Part model, mm, in its own coordinate system. A direction names the side the tool comes from. Coordinates: 2 decimals unless noted, no trailing zeros. Order: outer loops, then holes, each group sorted by start corner. A loop starts at its lowest first (then second) coordinate and runs counter-clockwise, first axis right, second up. Notation, with made-up numbers: M 75.5,6 L 90.5,6 A19 ccw 90.5,19 Z; hole C 28,-36 d2. An arc over 180 degrees is marked long. Answer in a Markdown table with one row per item. Add a question column.
from build123d import *

# Parameters (mm, degrees)
SKETCH1_W                     = 64.008
SKETCH1_H                     = 24.9936
BOSS_EXTRUDE1_DEPTH           = 6.35
SKETCH2_W                     = 64.008
SKETCH2_H                     = 6.35
BOSS_EXTRUDE2_DEPTH           = 82.55
CBORE_FOR_M5_SHCS1_AT_2_COUNT = 2
CBORE_FOR_M5_SHCS1_AT_2_PITCH = 50
SKETCH8_W                     = 10.414
SKETCH8_H                     = 82.55
CUT_EXTRUDE1_DEPTH            = 112.120735621
SKETCH9_W                     = 3.048
SKETCH9_H                     = 82.55
CUT_EXTRUDE3_DEPTH            = 112.120735621


with BuildPart() as part:
    # Sketch1 → Boss-Extrude1 (new body)
    with BuildSketch(Plane.XY):
        with Locations((32.004, 12.4968)):
            Rectangle(SKETCH1_W, SKETCH1_H)
    extrude(amount=BOSS_EXTRUDE1_DEPTH)

    # Sketch2 → Boss-Extrude2 (add)
    with BuildSketch(Plane.XY.offset(6.35)):
        with Locations((32.004, 3.175)):
            Rectangle(SKETCH2_W, SKETCH2_H)
    extrude(amount=BOSS_EXTRUDE2_DEPTH)

    # Sketch7 → CBORE for M5 SHCS1 (revolve, cut)
    with BuildSketch(Plane(origin=(7, 12.5, 6.35), x_dir=(0, -1, 0), z_dir=(1, 0, 0))):
        Polygon((0, 0), (0, 6.35), (2.75, 6.35), (2.75, 5), (5, 5), (5, 0.025), (5.025, 0), align=None)
    cbore_for_m5_shcs1 = revolve(axis=Axis((7, 12.5, 12.7), (0, 0, -1)), mode=Mode.SUBTRACT)

    # CBORE for M5 SHCS1 at 2: CBORE for M5 SHCS1 ×2
    with Locations(*[(i * CBORE_FOR_M5_SHCS1_AT_2_PITCH, 0, 0) for i in range(1, CBORE_FOR_M5_SHCS1_AT_2_COUNT)]):
        add(cbore_for_m5_shcs1, mode=Mode.SUBTRACT)

    # Sketch8 → Cut-Extrude1 (cut, through all)
    with BuildSketch(Plane(origin=(0, 6.35, 0), x_dir=(1, 0, 0), z_dir=(0, 1, 0))):
        with Locations((5.207, -47.625)):
            Rectangle(SKETCH8_W, SKETCH8_H)
    extrude(amount=-CUT_EXTRUDE1_DEPTH, mode=Mode.SUBTRACT)

    # Sketch9 → Cut-Extrude3 (cut, through all)
    with BuildSketch(Plane(origin=(0, 6.35, 0), x_dir=(1, 0, 0), z_dir=(0, 1, 0))):
        with Locations((62.484, -47.625)):
            Rectangle(SKETCH9_W, SKETCH9_H)
    extrude(amount=-CUT_EXTRUDE3_DEPTH, mode=Mode.SUBTRACT)


solid = part.part
(1) Slice it at D-D (x = 7). List the corners of the cut face in (y, z) (3 decimals).
(2) Slice it at B-B (y = 12.5). List the corners of the cut face in (x, z) (3 decimals), and give its area (3 significant figures).
(3) Pull direction Y, two halves, no side cores. Call faces 5 (the flat face through (39, 0, 44)), 6 (the cylindrical face through (52.784, 9.812, 3.872)), 7 (the flat face through (0, 12, 3)): pulls with the +Y half, pulls with the -Y half, needs draft (parallel to the pull), parting line crosses it, or undercut.
(4) 3-axis set-ups, long thin cutter, end or side, ignore diameter. For faces 1 (the flat face through (35, 6.35, 47)), 2 (the flat face through (60.96, 3, 48)), 3 (the flat face through (10.414, 3, 48)), 4 (the cylindrical face through (5.5, 7.73, 3.87)): which of +Z, -Z, +X, -X, +Y, -Y reach the whole face in a straight line?
(5) Wall check: line 1 (X direction, y = 12.5, z = 3.85); line 2 (X direction, y = 12.5, z = 0.85); line 3 (Y direction, x = 7, z = 4). Give the ranges that are in metal, low to high.
(6) Drop flat-ended pins along their axis: P1, Ø5, axis at x = 10, y = 13, coming from the -Z side; P2, Ø6, axis at x = 57, y = 12.5, coming from the +Z side; P3, Ø7, axis at y = 2.5, z = 39.5, coming from the +X side; P4, Ø8, axis at x = 5.5, y = 14.5, coming from the +Z side. Give the stop position or say it passes through.
(7) Slice it at A-A (x = 57). List the corners of the cut face in (y, z) (3 decimals).
(8) Slice it at C-C (y = 3.5). List the corners of the cut face in (x, z).
Computed:
| question | item | result |
|---|---|---|
| 1 | outline | M 0,0 L 9.75,0 L 9.75,1.35 L 7.5,1.35 L 7.5,6.325 L 7.475,6.35 L 0,6.35 Z; M 15.25,0 L 24.994,0 L 24.994,6.35 L 17.525,6.35 L 17.5,6.325 L 17.5,1.35 L 15.25,1.35 Z |
| 2 | outline | M 0,0 L 4.25,0 L 4.25,1.35 L 2,1.35 L 2,6.325 L 1.975,6.35 L 0,6.35 Z; M 9.75,0 L 54.25,0 L 54.25,1.35 L 52,1.35 L 52,6.325 L 51.975,6.35 L 12.025,6.35 L 12,6.325 L 12,1.35 L 9.75,1.35 Z; M 59.75,0 L 64.008,0 L 64.008,6.35 L 62.025,6.35 L 62,6.325 L 62,1.35 L 59.75,1.35 Z |
| 2 | area | 292 mm^2 |
| 3 | face 5 | pulls with the -Y half |
| 3 | face 6 | undercut |
| 3 | face 7 | needs draft |
| 4 | face 1 | +Z, +X, -X, +Y |
| 4 | face 2 | +Z, +X, +Y, -Y |
| 4 | face 3 | +Z, -X, +Y, -Y |
| 4 | face 4 | +Z |
| 5 | line 1 | x = 0 to 2, 12 to 52, 62 to 64.01 |
| 5 | line 2 | x = 0 to 4.25, 9.75 to 54.25, 59.75 to 64.01 |
| 5 | line 3 | y = 0 to 7.5, 17.5 to 24.99 |
| 6 | P1 | stops at z = 0 |
| 6 | P2 | stops at z = 1.35 |
| 6 | P3 | stops at x = 60.96 |
| 6 | P4 | stops at z = 6.35 |
| 7 | outline | M 0,0 L 9.75,0 L 9.75,1.35 L 7.5,1.35 L 7.5,6.325 L 7.475,6.35 L 6.35,6.35 L 6.35,88.9 L 0,88.9 Z; M 15.25,0 L 24.994,0 L 24.994,6.35 L 17.525,6.35 L 17.5,6.325 L 17.5,1.35 L 15.25,1.35 Z |
| 8 | outline | M 0,0 L 64.01,0 L 64.01,6.35 L 60.96,6.35 L 60.96,88.9 L 10.41,88.9 L 10.41,6.35 L 0,6.35 Z |
